Answer from the drawing. Dimensions are ordinates in mm from the lowest x, y and z of the part. Give positions to 0.01 mm unless a question says otherwise; leave off trailing zeros. Write each loop counter-clockwise with the first axis right and the second up, starting at its lowest first coordinate (ties: lowest second). Pieces come first, ordered by that corner, then holes. Notation, with made-up numbers: M -3.75,83 L 40.25,83 A26 ccw 40.25,102 Z; hole C 78.5,4 d1. An arc over 180 degrees is marked long. Answer as a JSON object with one key per item and string values.
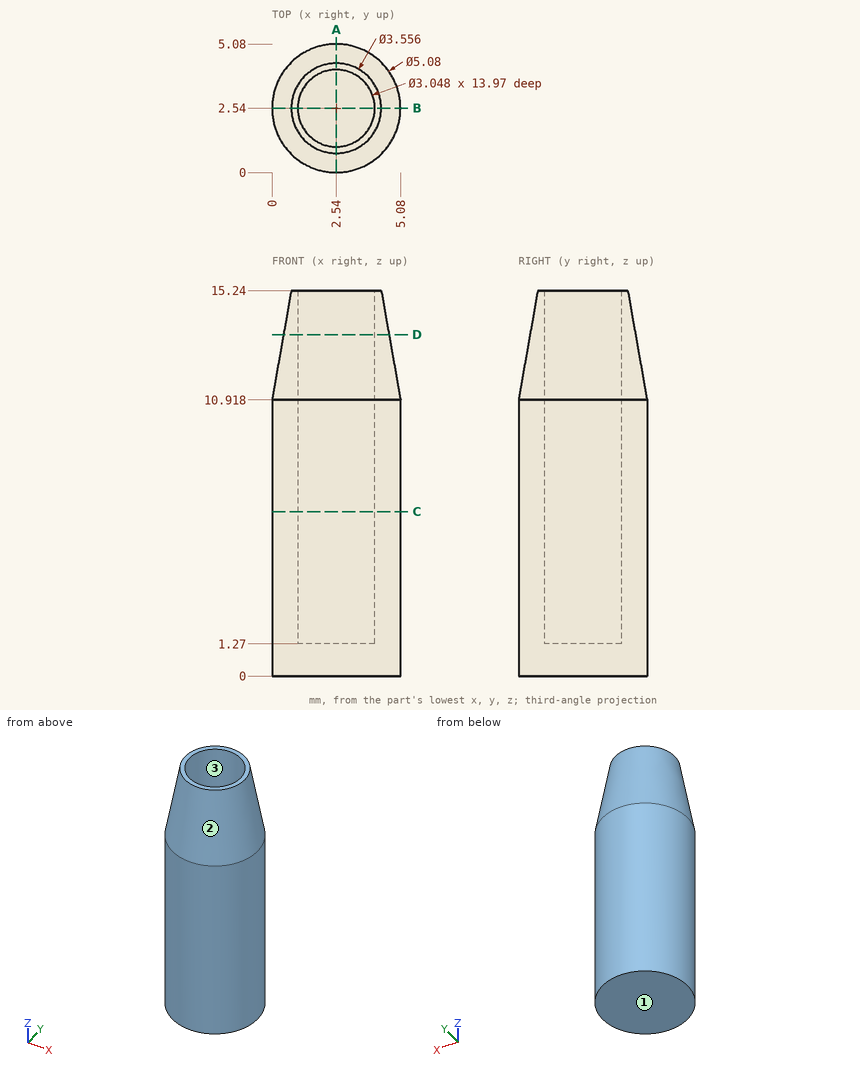
1. Consider line 1 along Y through (x, z) = (2.54, 10.5); line 2 along Z through (x, y) = (2.8, 2.45); line 3 along X through (y, z) = (2.85, 12.5). Determine where each line is inside the solid, lowest interval first.
Verdict:
{"line 1": "y = 0 to 1.02, 4.06 to 5.08", "line 2": "z = 0 to 1.27", "line 3": "x = 0.3 to 1.05, 4.03 to 4.78"}
2. A cutting plane is placed at D-D, the plane z = 13.5. Give the vertices of the cut face in (x, y) (1 decimal).
Verdict:
{"outline": "C 2.5,2.5 d4.2; hole C 2.5,2.5 d3"}
3. A cutting plane is placed at C-C, the plane z = 6.5. Give the vertices of the cut face in (x, y).
Verdict:
{"outline": "C 2.54,2.54 d5.08; hole C 2.54,2.54 d3.05"}
4. The mould has two halves that part along X. Classify the marked faces 1, 2 and 3: released by +X, released by -X, zero draft, split by the parting line, or undercut.
Verdict:
{"face 1": "zero draft", "face 2": "split by the parting line", "face 3": "undercut"}
5. A cutting plane is placed at A-A, the plane x = 2.54. Give the vertices of the cut face in (y, z).
Verdict:
{"outline": "M 0,0 L 5.08,0 L 5.08,10.92 L 4.32,15.24 L 4.06,15.24 L 4.06,1.27 L 1.02,1.27 L 1.02,15.24 L 0.76,15.24 L 0,10.92 Z"}
